from build123d import *

# Parameters (mm, degrees)
SKETCH1_R           = 0.8509
BOSS_EXTRUDE3_DEPTH = 3.175


with BuildPart() as part:
    # Sketch1 → Boss-Extrude3 (new body)
    # profile 1 of 2: a face of its own
    with BuildSketch(Plane(origin=(0, 0, 0), x_dir=(1, 0, 0), z_dir=(0, 1, 0))):
        with BuildLine():
            Line((-26.618355099, 139.499410737), (-12.357546713, 104.145756125))
            ThreePointArc((-12.357546713, 104.145756125), (-11.974349365, 102.985269848), (-11.743579527, 101.785139069))
            Line((-11.743579527, 101.785139069), (-7.99527824, 72.072064446))
            ThreePointArc((-7.99527824, 72.072064446), (-7.946716363, 71.409174189), (-7.967711413, 70.744839217))
            Line((-7.967711413, 70.744839217), (-13.823023592, 1.163211045))
            ThreePointArc((-13.823023592, 1.163211045), (-0.322101588, -13.868139447), (13.862122414, 0.520195482))
            Line((13.862122414, 0.520195482), (11.138065029, 73.110631708))
            Line((11.138065029, 73.110631708), (9.439411602, 118.376195482))
            ThreePointArc((9.439411602, 118.376195482), (9.128634942, 120.450134843), (8.367932415, 122.40439641))
            Line((8.367932415, 122.40439641), (-7.278206254, 150.703639796))
            ThreePointArc((-7.278206254, 150.703639796), (-21.808106397, 153.490299925), (-26.618355099, 139.499410737))
        make_face()
        with Locations(Location((0, 0, 0), (0, 0, 270))):
            Circle(SKETCH1_R, mode=Mode.SUBTRACT)
        with Locations(Location((0, 118.021968393, 0), (0, 0, 270))):
            Circle(SKETCH1_R, mode=Mode.SUBTRACT)
        with Locations(Location((-16.149303345, 143.722372767, 0), (0, 0, 270))):
            Circle(SKETCH1_R, mode=Mode.SUBTRACT)
        with BuildLine():
            ThreePointArc((-2.955223154, 72.707866873), (-2.867811775, 71.514664411), (-2.905602865, 70.318861461))
            Line((-2.905602865, 70.318861461), (-7.652524964, 13.908791704))
            ThreePointArc((-7.652524964, 13.908791704), (0.876701263, 15.850773479), (9.139736464, 12.98001704))
            Line((9.139736464, 12.98001704), (5.991360589, 96.877654221))
            Line((5.991360589, 96.877654221), (-5.816334076, 95.388114762))
            Line((-5.816334076, 95.388114762), (-2.955223154, 72.707866873))
        make_face(mode=Mode.SUBTRACT)
    # profile 2 of 2: a face of its own
    with BuildSketch(Plane(origin=(0, 0, 0), x_dir=(1, 0, 0), z_dir=(0, 1, 0))):
        with BuildLine():
            Line((7.71861106, 50.850039017), (-2.955223154, 72.707866873))
            ThreePointArc((-2.955223154, 72.707866873), (-2.867811775, 71.514664411), (-2.905602865, 70.318861461))
            Line((-2.905602865, 70.318861461), (-3.260786549, 66.098034587))
            Line((-3.260786549, 66.098034587), (8.012738289, 43.012163072))
            Line((8.012738289, 43.012163072), (7.71861106, 50.850039017))
        make_face()
    extrude(amount=BOSS_EXTRUDE3_DEPTH)


solid = part.part
Source: CAD feature listing. Evaluate the final solid. Frame: model axes, mm. A direction names the side the tool comes from. Give positions to 0.01 mm unless a question says otherwise; leave off trailing zeros. Order: outer loops, then holes, each group sorted by start corner. A loop starts at its lowest first (then second) coordinate and runs counter-clockwise, first axis right, second up. Notation, with made-up numbers: (-11, 20.25) -> (-2, 20.25) arc R33 cw to (-2, 53.25) -> close; hole circle Ø2 at (70.5, -15.75). An arc over 180 degrees is marked (long way). Use a Markdown table: item, result.
1) Section query D-D, the plane x = -20. Return the cut outline in (y, z) (3 decimals).
Answer list:
| item | result |
|---|---|
| outline | (0, -154.334) -> (3.175, -154.334) -> (3.175, -123.092) -> (0, -123.092) -> close |
2) Section query A-A, the plane z = -58. Return the cut outline in (x, y) (3 decimals).
Answer list:
| item | result |
|---|---|
| outline | (-9.04, 0) -> (-3.942, 0) -> (-3.942, 3.175) -> (-9.04, 3.175) -> close; (0.694, 0) -> (4.227, 0) -> (4.227, 3.175) -> (0.694, 3.175) -> close; (7.45, 0) -> (11.705, 0) -> (11.705, 3.175) -> (7.45, 3.175) -> close |
3) Section query C-C, the plane y = 1.1. Return the cut outline in (x, z) (3 decimals).
Answer list:
| item | result |
|---|---|
| outline | (-26.618, -139.499) arc R11.289 ccw to (-7.278, -150.704) -> (8.368, -122.404) arc R9.446 ccw to (9.439, -118.376) -> (13.862, -0.52) arc R13.872 ccw (long way) to (-13.823, -1.163) -> (-7.968, -70.745) arc R6.35 cw to (-7.995, -72.072) -> (-11.744, -101.785) arc R9.483 cw to (-12.358, -104.146) -> close; hole circle Ø1.702 at (-16.149, -143.722); hole (-7.653, -13.909) -> (-3.261, -66.098) -> (8.013, -43.012) -> (9.14, -12.98) arc R15.875 cw to start; hole (-5.816, -95.388) -> (5.991, -96.878) -> (7.719, -50.85) -> (-2.955, -72.708) -> close; hole circle Ø1.702 at (0, -118.022); hole circle Ø1.702 at (0, 0) |
4) Ray query, line 1 along X through (y, z) = (1.15, 0); line 2 along Z through (x, y) = (-1.5, 0.85); line 3 along X through (y, z) = (0.45, -61.5). Return the intervals inside material, ascending. Write a range as [from, to].
Answer list:
| item | result |
|---|---|
| line 1 | [-13.87, -0.85], [0.85, 13.87] |
| line 2 | [-140.25, -95.93], [-69.73, -62.49], [-15.8, 13.79] |
| line 3 | [-8.75, -3.65], [-1.02, 2.52], [7.32, 11.57] |
5) Mould query, pull axis Z, two halves, no side actions, for faces 1 (the flat face through (2.297, 1.565, -54.717)), 2 (the flat face through (-7, 3.175, -72)), 3 (the flat face through (0.65, 1.57, -136.36)). Classes: +Z half, -Z half, draft (parallel to the pull), parting line (faces both ways), or undercut.
Answer list:
| item | result |
|---|---|
| face 1 | undercut |
| face 2 | draft |
| face 3 | -Z half |
6) Section query B-B, the plane x = 4. Return the cut outline in (y, z) (3 decimals), then the cut area to 3 significant figures.
Answer list:
| item | result |
|---|---|
| outline | (0, -130.305) -> (3.175, -130.305) -> (3.175, -96.626) -> (0, -96.626) -> close; (0, -58.465) -> (3.175, -58.465) -> (3.175, -51.229) -> (0, -51.229) -> close; (0, -15.363) -> (3.175, -15.363) -> (3.175, 13.283) -> (0, 13.283) -> close |
| area | 221 mm² |
7) Reachability of faces 4 (the flat face through (0.17, 1.565, -96.143)), 5 (the flat face through (-9.896, 1.565, -87.137)), 6 (the flat face through (-7, 0, -72)) from +Z, -Z, +X, -X, +Y, -Y: full face, straight path, thin tool, end or side. Return the list, or none.
Answer list:
| item | result |
|---|---|
| face 4 | +Y, -Y |
| face 5 | -X, +Y, -Y |
| face 6 | +Z, -Z, +X, -X, -Y |
8) Contact query for flat-ended pins moving along their axis: P1, Ø1, axis at x = 7, z = -22.5, coming from the -Y side; P2, Ø1.5, axis at x = -14, y = 0.5, coming from the -Z side; P3, Ø12, axis at x = -3.5, z = -111.5, coming from the -Y side; P4, Ø1.5, axis at y = 0.5, z = -26, coming from the +X side. Output: stop coordinate, or through.
Answer list:
| item | result |
|---|---|
| P1 | through |
| P2 | z = -154.92 |
| P3 | y = 0 |
| P4 | x = 12.93 |
